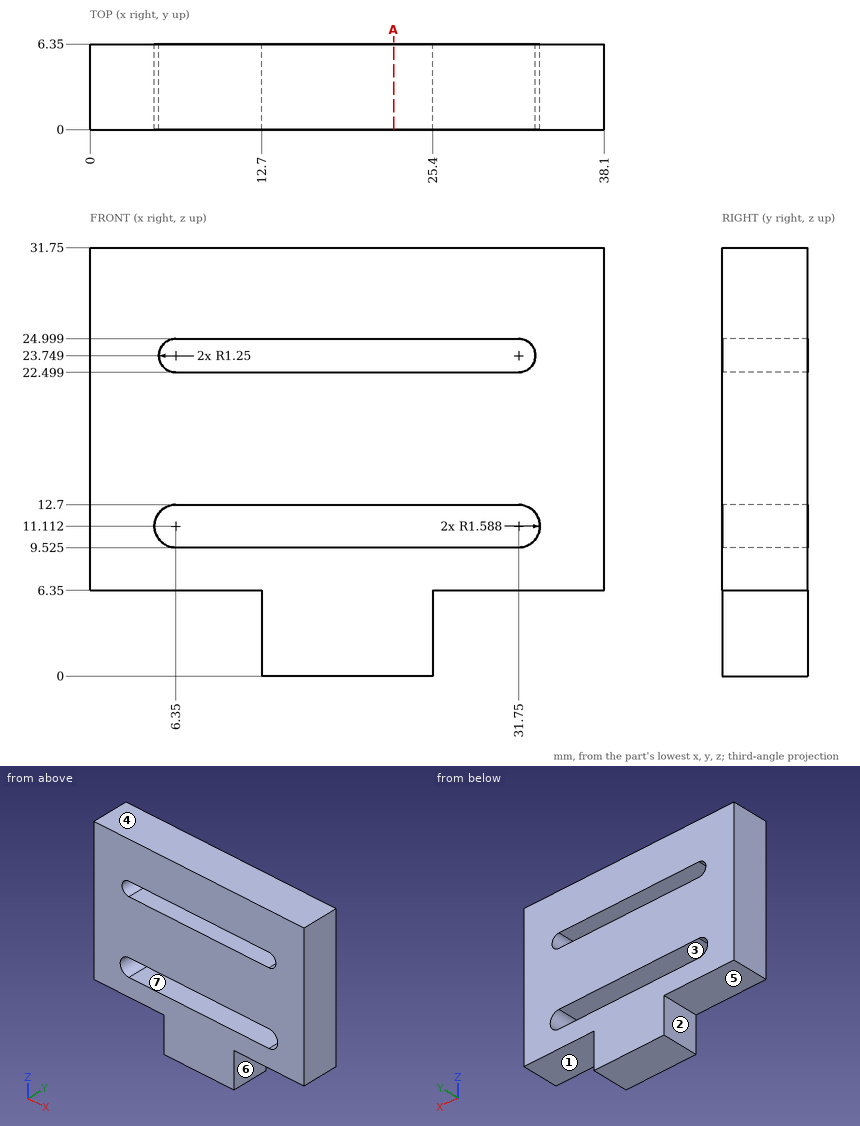
Can you work these out from the drawing? Everything is in mm from the part's minimum corner. A direction names the side the tool comes from. Give positions to 0.01 mm unless a question says otherwise; leave off trailing zeros. Return JSON: item names as keys, results as strings.
Item 1: We'd pull the mould along Z, two halves only. Please class the marked faces 1, 2 and 3: +Z half, -Z half, draft (parallel to the pull), parting line (faces both ways), or undercut.
Geometry results:
{"face 1": "-Z half", "face 2": "draft", "face 3": "undercut"}
Item 2: Which directions (+Z, -Z, +X, -X, +Y, -Y) give clear straight access to the entire face, cutting with the end or side of a thin tool? Please do the marked faces 4, 5, 6 and 7.
Geometry results:
{"face 4": "+Z, +X, -X, +Y, -Y", "face 5": "-Z, -X, +Y, -Y", "face 6": "-Z, +X, +Y, -Y", "face 7": "+Y, -Y"}
Item 3: If we section it at A-A on x = 22.5: Count the separate pieces of the cut face and the enclosed holes in it.
Geometry results:
{"separate pieces": "3", "enclosed holes": "0"}
Item 4: I need wall thicknesses on L1, parallel to Z at x = 34.5, y = 4; L2, parallel to X at y = 5.5, z = 3.5; L3, parallel to X at y = 4.5, z = 11.5. Which ranges of each line are inside material? Lowest first, please. Write a range as from..to.
Geometry results:
{"L1": "z = 6.35..31.75", "L2": "x = 12.7..25.4", "L3": "x = 0..4.81, 33.29..38.1"}
Item 5: I'm going to push flat-ended pins straight in: pin 1 (1.9 mm diameter, centred on y = 4, z = 2.5, fed in from -X); pin 2 (1.5 mm diameter, centred on x = 31, y = 1, fed in from -Z). Where does each tip first touch, or does it pass through?
Geometry results:
{"pin 1": "stops at x = 12.7", "pin 2": "stops at z = 6.35"}
